Could you check a few things on this model? Use its own coordinates, in mm. A direction names the side the tool comes from. Give positions to 0.01 mm unless a question says otherwise; leave off trailing zeros. Write each loop counter-clockwise with the first axis right and the second up, starting at its lowest first coordinate (ties: lowest second). Pieces come first, ordered by that corner, then holes. Notation, with made-up numbers: (67, 58) - (121, 58) arc R14 ccw to (121, 62) - close; hole circle Ø9 at (73.25, 26.5). An arc over 180 degrees is marked (long way). Answer in a Markdown table with one row per item.
from build123d import *

# Parameters (mm, degrees)
SKETCH_1_R      = 10
EXTRUDE_1_DEPTH = 20


with BuildPart() as part:
    # 草图1 → 凸台-拉伸1 (new body)
    with BuildSketch(Plane.XY.offset(-35.913663537)):
        with BuildLine():
            Line((-92.03956228, 673.590403503), (-39.698813198, 709.260436791))
            ThreePointArc((-39.698813198, 709.260436791), (-18.856217474, 705.312500182), (-22.804154083, 684.469904458))
            Line((-22.804154083, 684.469904458), (-75.144903165, 648.799871169))
            ThreePointArc((-75.144903165, 648.799871169), (-95.98749889, 652.747807779), (-92.03956228, 673.590403503))
        make_face()
        with Locations((-31.251483641, 696.865170625)):
            Circle(SKETCH_1_R, mode=Mode.SUBTRACT)
        with BuildLine():
            Line((-74.722353088, 665.813062766), (-92.462112357, 665.813062766))
            ThreePointArc((-92.462112357, 665.813062766), (-83.592232723, 651.195137336), (-74.722353088, 665.813062766))
        make_face(mode=Mode.SUBTRACT)
    extrude(amount=EXTRUDE_1_DEPTH)


solid = part.part
1) Imagine slicing it at B-B (z = -21.25). List the corners of the cut face in (x, y) for me, then the cut area to 3 significant figures.
Check values:
| item | result |
|---|---|
| outline | (-92.04, 673.59) arc R15 ccw to (-75.14, 648.8) - (-22.8, 684.47) arc R15 ccw to (-39.7, 709.26) - close; hole (-92.46, 665.81) arc R10 ccw (long way) to (-74.72, 665.81) - close; hole circle Ø20 at (-31.25, 696.87) |
| area | 2,050 mm2 |
2) On a 3-axis mill with a long thin cutter (end or side, diameter ignored), from which of +Z, -Z, +X, -X, +Y, -Y can I reach the whole of each face in a straight line? I mean faces 1 (the face through (-83, 665.813, -26)), 2 (the face through (-57, 679, -35.914)). Say none if no direction works.
Check values:
| item | result |
|---|---|
| face 1 | +Z, -Z |
| face 2 | -Z, +X, -X, +Y, -Y |
3) Imagine slicing it at D-D (y = 682). List the corners of the cut face in (x, z) for me, then the cut area to 3 significant figures.
Check values:
| item | result |
|---|---|
| outline | (-79.7, -35.91) - (-26.43, -35.91) - (-26.43, -15.91) - (-79.7, -15.91) - close |
| area | 1,070 mm2 |
4) If I drill on line 1 (Y direction, x = -36, z = -26.25); line 2 (X direction, y = 692, z = -31); line 3 (X direction, y = 699.5, z = -32), over which ranges is the centre line in solid material (lowest first)?
Check values:
| item | result |
|---|---|
| line 1 | y = 675.48 to 688.06, 705.67 to 711.09 |
| line 2 | x = -65.03 to -39.99, -22.51 to -17.06 |
| line 3 | x = -54.02 to -40.9, -21.6 to -16.48 |
5) We'd pull the mould along Y, two halves only. Please class faces 3 (the face through (-66.2, 691.2, -26.1)), 4 (the face through (-57, 679, -15.914)), 5 (the face through (-26.64, 687.99, -26.05)), 6 (the face through (-48.608, 666.885, -26.054)): +Y half, -Y half, draft (parallel to the pull), parting line (faces both ways), or undercut.
Check values:
| item | result |
|---|---|
| face 3 | +Y half |
| face 4 | draft |
| face 5 | undercut |
| face 6 | -Y half |
6) Will these pins go through, and if not, where does the flat tip stop? P1, Ø5, axis at x = -47, z = -23.5, coming from the -Y side; P2, Ø1, axis at y = 673, z = -28.5, coming from the -X side; P3, Ø3, axis at y = 682.5, z = -19, coming from the -X side.
Check values:
| item | result |
|---|---|
| P1 | stops at y = 666.28 |
| P2 | stops at x = -93.45 |
| P3 | stops at x = -81.17 |
7) Imagine slicing it at A-A (x = -26). List the corners of the cut face in (y, z) for me, then the cut area to 3 significant figures.
Check values:
| item | result |
|---|---|
| outline | (682.29, -35.91) - (688.36, -35.91) - (688.36, -15.91) - (682.29, -15.91) - close; (705.38, -35.91) - (710.92, -35.91) - (710.92, -15.91) - (705.38, -15.91) - close |
| area | 232 mm2 |
8) Imagine slicing it at C-C (y = 699.5). List the corners of the cut face in (x, z) for me.
Check values:
| item | result |
|---|---|
| outline | (-54.02, -35.91) - (-40.9, -35.91) - (-40.9, -15.91) - (-54.02, -15.91) - close; (-21.6, -35.91) - (-16.48, -35.91) - (-16.48, -15.91) - (-21.6, -15.91) - close |
